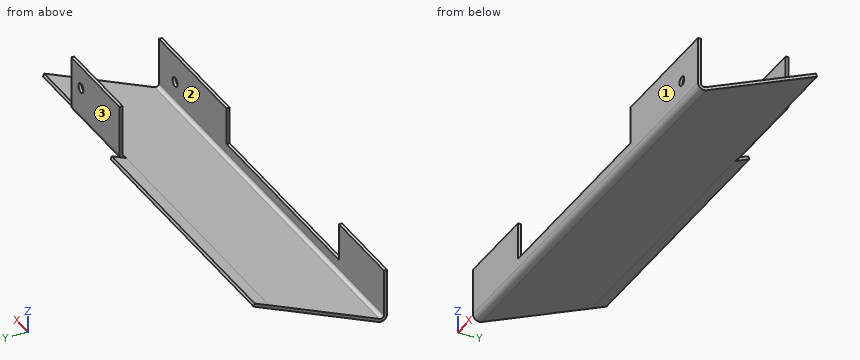
```python
from build123d import *

# Parameters (mm, degrees)
T_LE_DE_BASE_PLI_E1_DEPTH = 140
ESQUISSE6_W               = 70
ESQUISSE6_H               = 12
ENL_V_MAT_EXTRU_1_DEPTH   = 1
ESQUISSE7_W               = 90
ESQUISSE7_H               = 8.077316225
ESQUISSE7_W_2             = 20
ENL_V_MAT_EXTRU_2_DEPTH   = 148.230392024
ESQUISSE8_W               = 89
ESQUISSE8_H               = 5
PATTE1_DEPTH              = 1
ESQUISSE11_R              = 1.5
ENL_V_MAT_EXTRU_3_DEPTH   = 1
ESQUISSE12_R              = 1.5
ENL_V_MAT_EXTRU_4_DEPTH   = 1


# Sheet-metal steps are written as plain solids
with BuildPart() as part:
    # Esquisse1 → Tôle de base pliée1 (new body)
    with BuildSketch(Plane(origin=(0, 0, 0), x_dir=(0, 0, -1), z_dir=(1, 0, 0))):
        with BuildLine():
            Line((0, 0), (14.997077996, 0))
            ThreePointArc((14.997077996, 0), (16.661676799, 0.891347294), (16.842539964, 2.770889177))
            Line((16.842539964, 2.770889177), (2.01342604, 38.270889177))
            ThreePointArc((2.01342604, 38.270889177), (1.276616778, 39.164598804), (0.167964072, 39.5))
            Line((0.167964072, 39.5), (-16, 39.5))
            Line((-16, 39.5), (-16, 38.5))
            Line((-16, 38.5), (0.167964072, 38.5))
            ThreePointArc((0.167964072, 38.5), (0.722290425, 38.332299402), (1.090695056, 37.885444588))
            Line((1.090695056, 37.885444588), (15.91980898, 2.385444588))
            ThreePointArc((15.91980898, 2.385444588), (15.829377397, 1.445673647), (14.997077996, 1))
            Line((14.997077996, 1), (0, 1))
            Line((0, 1), (0, 0))
        make_face()
    extrude(amount=-T_LE_DE_BASE_PLI_E1_DEPTH)

    # Esquisse6 → Enlèv. mat.-Extru.1 (cut)
    with BuildSketch(Plane.XZ):
        with Locations((-77, -6)):
            Rectangle(ESQUISSE6_W, ESQUISSE6_H)
    extrude(amount=-ENL_V_MAT_EXTRU_1_DEPTH, mode=Mode.SUBTRACT)

    # Esquisse7 → Enlèv. mat.-Extru.2 (cut, through all)
    with BuildSketch(Plane(origin=(0, 6.401909959, -15.325784447), x_dir=(-1, 0, 0), z_dir=(0, 0.38544458835969, -0.9227309842550152))):
        with Locations((95, 38.57632918)):
            Rectangle(ESQUISSE7_W, ESQUISSE7_H)
        with Locations((10, 38.57632918)):
            Rectangle(ESQUISSE7_W_2, ESQUISSE7_H)
    extrude(amount=-ENL_V_MAT_EXTRU_2_DEPTH, mode=Mode.SUBTRACT)

    # Esquisse8 → Patte1 (add)
    with BuildSketch(Plane(origin=(0, 6.401909959, -15.325784447), x_dir=(-1, 0, 0), z_dir=(0, 0.38544458835969003, -0.9227309842550152))):
        with Locations((95.5, 37.037671067)):
            Rectangle(ESQUISSE8_W, ESQUISSE8_H)
    extrude(amount=-PATTE1_DEPTH)

    # Esquisse11 → Enlèv. mat.-Extru.3 (cut)
    with BuildSketch(Plane(origin=(0, 1, 0), x_dir=(1, 0, 0), z_dir=(0, 1, 0))):
        with Locations(Location((-10, 9, 0), (0, 0, 270))):
            Circle(ESQUISSE11_R)
    extrude(amount=-ENL_V_MAT_EXTRU_3_DEPTH, mode=Mode.SUBTRACT)

    # Esquisse12 → Enlèv. mat.-Extru.4 (cut)
    with BuildSketch(Plane(origin=(0, 39.5, 0), x_dir=(1, 0, 0), z_dir=(0, 1, 0))):
        with Locations(Location((-26, -9, 0), (0, 0, 270))):
            Circle(ESQUISSE12_R)
    extrude(amount=-ENL_V_MAT_EXTRU_4_DEPTH, mode=Mode.SUBTRACT)


solid = part.part
```
Verification items for the finished model (mm, model axes). Face numbers are marked on the shaded views. Coordinates: 2 decimals unless noted, no trailing zeros. Loops run counter-clockwise (first coordinate to the right, second up) from the corner with the lowest first, then second, coordinate; pieces in that order, holes last. Notation, with made-up numbers: (-5.75, 45.5) - (12.25, 45.5) arc R12 cw to (12.25, 49.5) - close; hole circle Ø2 at (75, 18). An arc over 180 degrees is marked (long way). Return JSON: item names as keys, results as strings.
1. Thickness scan on L1, parallel to X at y = 0.35, z = -9; L2, parallel to X at y = 38.85, z = 9; L3, parallel to Y at x = -41.5, z = -6.5. Record the ranges inside material, lowest first.
Established:
{"L1": "x = -140 to -112, -42 to -11.5, -8.5 to 0", "L2": "x = -50 to -27.5, -24.5 to -20", "L3": "y = 0 to 1, 24.94 to 27.53"}
2. Section check C-C, the plane z = -3.5. Record the boundary of the cut face in (x, y), then the cut area to 3 significant figures.
Established:
{"outline": "(-140, 0) - (-112, 0) - (-112, 1) - (-140, 1) - close; (-140, 32.12) - (0, 32.12) - (0, 34.71) - (-140, 34.71) - close; (-42, 0) - (0, 0) - (0, 1) - (-42, 1) - close", "area": "433 mm2"}
3. Section check A-A, the plane x = -10. Record the boundary of the cut face in (y, z).
Established:
{"outline": "(0, -15) arc R2 ccw to (2.77, -16.84) - (38.27, -2.01) - (37.89, -1.09) - (2.39, -15.92) arc R1 cw to (1, -15) - (1, -10.5) - (0, -10.5) - close; (0, -7.5) - (1, -7.5) - (1, 0) - (0, 0) - close"}
4. Mould release check, pull along Y, two halves, no side actions. Record for the marked faces 1, 2 and 3: +Y half, -Y half, draft (parallel to the pull), parting line (faces both ways), or undercut.
Established:
{"face 1": "-Y half", "face 2": "undercut", "face 3": "+Y half"}
5. Go/stop test with flat-tipped pins: pin 1 (2.5 mm diameter, centred on y = 41, z = -0.5, fed in from +X); pin 2 (2.5 mm diameter, centred on x = -10, z = -9, fed in from -Y); pin 3 (1 mm diameter, centred on x = -47.5, z = 9.5, fed in from +Y). Record where each tip stops, or that it passes through.
Established:
{"pin 1": "stops at x = -51", "pin 2": "stops at y = 15.96", "pin 3": "stops at y = 39.5"}
6. Section check B-B, the plane z = 9. Record the boundary of the cut face in (x, y), then the cut area to 3 significant figures.
Established:
{"outline": "(-50, 38.5) - (-27.5, 38.5) - (-27.5, 39.5) - (-50, 39.5) - close; (-24.5, 38.5) - (-20, 38.5) - (-20, 39.5) - (-24.5, 39.5) - close", "area": "27.0 mm2"}
7. Section check D-D, the plane x = -70. Record the boundary of the cut face in (y, z).
Established:
{"outline": "(0, -15) arc R2 ccw to (2.77, -16.84) - (42.88, -0.09) - (42.5, 0.84) - (2.39, -15.92) arc R1 cw to (1, -15) - (1, -12) - (0, -12) - close"}
